Autodesk Inventor part; units mm, degrees
ref_plane "Work Plane1" through (0, 0, -15) normal (0, 0, 1) x (1, 0, 0)
ref_plane "YZ Plane" through (0, 0, 0) normal (1, 0, 0) x (0, 1, 0)
ref_plane "XZ Plane" through (0, 0, 0) normal (0, 1, 0) x (-1, 0, 0)
sketch "Sketch1" plane through (0, 0, 0) normal (0, 0, 1) x (1, 0, 0)
  line L0 (0, 0) -> (25, 0)
  line L1 (25, 0) -> (25, 40)
  line L2 (25, 40) -> (0, 40)
  line L3 (0, 40) -> (0, 0)
  dimension "d1" = 25
  dimension "d2" = 40
  dimension "d3" = 25
extrude "Extrusion1" add sketch "Sketch1" against normal blind 30
sketch "Sketch2" plane through (25, 0, 0) normal (1, 0, 0) x (0, 0, -1)
  line L0 (0, 0) -> (30, 0)
  circle A0 centre (15, 6.56) radius 2.46
extrude "Extrusion2" cut sketch "Sketch2" against normal blind 30
sketch "Sketch3" plane through (0, 0, 0) normal (-1, 0, 0) x (0, 0, 1)
  line L0 (0, 0) -> (-30, 0)
  line L1 (-25.05, 0) -> (-4.95, 0)
  line L2 (-4.95, 0) -> (-4.95, 33.12)
  line L3 (-4.95, 33.12) -> (-25.05, 33.12)
  line L4 (-25.05, 33.12) -> (-25.05, 0)
  dimension "d11" = 20.1
extrude "Extrusion3" cut sketch "Sketch3" against normal blind 20
sketch "Sketch4" plane through (0, 0, 0) normal (0, -1, 0) x (1, 0, 0)
  line L0 (20, -4.95) -> (20, -25.05)
  line L1 (20, -15) -> (25, -15)
  line L2 (25, 0) -> (25, -30)
  line L3 (20, -8.025) -> (25, -8.025)
  line L4 (25, -8.025) -> (25, -21.975)
  line L5 (25, -21.975) -> (20, -21.975)
  line L6 (20, -21.975) -> (20, -8.025)
  line L7 (20, -8.025) -> (25, -21.975) construction
  line L8 (25, -8.025) -> (20, -21.975) construction
  line L9 (25, -12.54) -> (25, -17.46)
  point P0 (0, 0)
  point P1 (22.5, -15)
  dimension "d14" = 13.95
extrude "Extrusion4" add sketch "Sketch4" along normal blind 15
sketch "Sketch5" plane through (20, 0, 0) normal (-1, 0, 0) x (0, 0, 1)
  circle A0 centre (-15, 6.56) radius 2.46
  circle A1 centre (-15, 6.56) radius 4.7025
  circle A2 centre (-15, 6.56) radius 2.46
  circle A3 centre (-15, 6.56) radius 2.46
  point P0 (0, 0)
  dimension "d17" = 9.405
extrude "Extrusion5" cut sketch "Sketch5" against normal blind 2.1
sketch "Sketch6" plane through (25, 0, 0) normal (1, 0, 0) x (0, 0, -1)
  circle A0 centre (15, 6.56) radius 4.7025
  line L0 (15, 6.56) -> (15, 23.56)
  circle A1 centre (15, 23.56) radius 2.46
  point P0 (0, 0)
  dimension "d20" = 17
  dimension "d21" = 4.92
extrude "Extrusion6" cut sketch "Sketch6" against normal blind 10 contours A1
sketch "Sketch7" plane through (20, 0, 0) normal (-1, 0, 0) x (0, 0, 1)
  circle A0 centre (-15, 23.56) radius 2.46
  circle A1 centre (-15, 23.56) radius 4.7025
  point P0 (0, 0)
  dimension "d24" = 9.405
extrude "Extrusion7" cut sketch "Sketch7" against normal blind 2.1
sketch "Sketch9" plane through (25, 0, 0) normal (1, 0, 0) x (0, 0, -1)
  circle A0 centre (15, 6.56) radius 2.46
  circle A1 centre (15, 6.56) radius 2.46
  circle A2 centre (15, 23.56) radius 2.46
  circle A3 centre (15, 23.56) radius 2.46
  line L0 (30, 40) -> (30, 0)
  line L1 (30, 0) -> (30, 40)
  line L2 (30, 40) -> (0, 40)
  line L3 (0, 40) -> (0, 0)
  line L4 (0, 0) -> (8.025, 0)
  line L5 (21.975, 0) -> (21.975, -15)
  line L6 (21.975, -15) -> (8.025, -15)
  line L7 (8.025, -15) -> (8.025, 0)
  line L8 (0, 0) -> (8.025, 0)
  line L9 (21.975, 0) -> (30, 0)
extrude "Extrusion8" add sketch "Sketch9" along normal blind 5
sketch "Sketch10" plane through (0, 40, 0) normal (0, 1, 0) x (1, 0, 0)
  line L0 (0, 30) -> (30, 30)
  line L1 (30, 0) -> (0, 0)
  line L2 (0, 30) -> (30, 30)
  line L3 (30, 30) -> (30, 0)
  line L4 (30, 0) -> (0, 0)
  line L5 (0, 0) -> (0, 30)
extrude "Extrusion9" add sketch "Sketch10" along normal blind 30
sketch "Sketch12" plane through (30, 0, 0) normal (1, 0, 0) x (0, 0, -1)
  circle A0 centre (15, 6.56) radius 2.46
  line L0 (15, 6.56) -> (15, 15.06)
  circle A1 centre (15, 15.06) radius 2.525
  point P0 (0, 0)
  dimension "d31" = 8.5
  dimension "d33" = 5.05
extrude "Extrusion10" cut sketch "Sketch12" against normal blind 30 contours A1
sketch "Sketch14" plane through (0, 0, 0) normal (0, 0, 1) x (1, 0, 0)
  line L0 (30, 70) -> (0, 70)
  line L1 (0, 70) -> (0, 85)
  line L2 (-15, 100) -> (-23, 100)
  line L3 (30, 0) -> (30, 70)
  line L4 (30, 122.5) -> (30, 70)
  arc A0 (0, 85) -> (-15, 100) centre (-15, 85) ccw
  line L5 (30, 105) -> (30, 100)
  line L6 (-23, 153) -> (15, 153)
  line L7 (-18, 150.5) -> (-23, 153)
  line L8 (-18, 102.5) -> (-23, 100)
  line L9 (-18, 102.5) -> (-13, 126.5)
  line L10 (-13, 126.5) -> (-18, 150.5)
  line L11 (30, 126.5) -> (15, 153)
  line L12 (30, 122.5) -> (30, 126.5)
  point P0 (0, 0)
  point P1 (0, 100)
  dimension "d47" = 30
  dimension "d54" = 15
extrude "Extrusion12" add sketch "Sketch14" against normal blind 30
sketch "Sketch15" plane through (0, 0, -25.05) normal (-1, 0, 0) x (0, 0, 1)
  line L0 (0, 33.12) -> (20.1, 33.12)
  line L1 (20.1, 33.12) -> (20.1, 0)
  line L2 (0, 33.12) -> (20.1, 33.12)
  line L3 (20.1, 33.12) -> (20.1, 31.1)
  line L4 (20.1, 31.1) -> (0, 31.1)
  line L5 (0, 31.1) -> (0, 33.12)
  point P0 (25.05, 0)
  dimension "d57" = 2.02
extrude "Extrusion13" add sketch "Sketch15" against normal blind 20
sketch "Sketch25" plane through (0, 0, 0) normal (0, 0, 1) x (1, 0, 0)
  line L0 (-15, 100) -> (-23, 100)
  line L1 (-15, 100) -> (-23, 100)
  line L2 (-23, 100) -> (-18, 102.5)
  line L3 (-23, 100) -> (-18, 102.5)
  line L4 (-18, 102.5) -> (-13, 126.5)
  line L5 (-18, 102.5) -> (-13, 126.5)
  line L6 (-13, 126.5) -> (-18, 150.5)
  line L7 (-13, 126.5) -> (-18, 150.5)
  line L8 (-18, 150.5) -> (-23, 153)
  line L9 (-18, 150.5) -> (-23, 153)
  line L10 (-23, 153) -> (15, 153)
  line L11 (-23, 153) -> (15, 153)
  line L12 (15, 153) -> (30, 126.5)
  line L13 (15, 153) -> (30, 126.5)
  line L14 (30, 126.5) -> (30, 76.5)
  line L15 (30, 0) -> (30, 126.5)
  line L16 (30, 76.5) -> (0, 76.5)
  arc A0 (0, 85) -> (-15, 100) centre (-15, 85) ccw
  line L17 (0, 76.5) -> (0, 85)
  line L18 (0, 85) -> (0, 0)
  arc A1 (0, 85) -> (-15, 100) centre (-15, 85) ccw
  dimension "d90" = 50
extrude "Extrusion14" add sketch "Sketch25" along normal blind 30
ref_plane "Work Plane1" through (0, 0, -15) normal (0, 0, 1) x (1, 0, 0)
mirror "Mirror1" about plane through (0, 0, -15) normal (0, 0, 1) of "Extrusion14"
properties part number "rec_a_48mm_x_90mm"
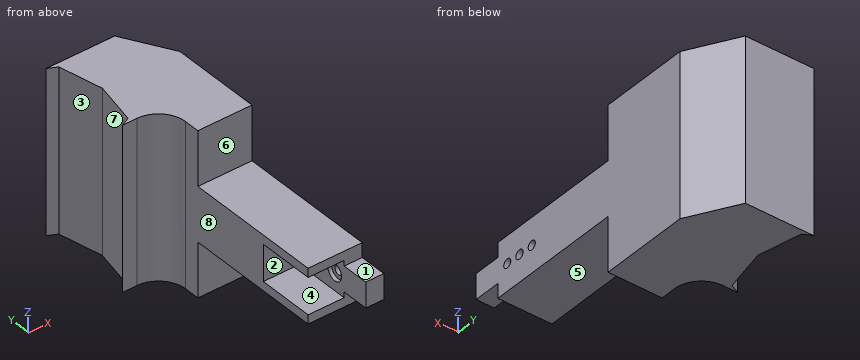
Here's how the part is built. I have some questions about the finished solid (model axes, mm). Face numbers are marked on the shaded views. A direction names the side the tool comes from. Give positions to 0.01 mm unless a question says otherwise; leave off trailing zeros. Order: outer loops, then holes, each group sorted by start corner. A loop starts at its lowest first (then second) coordinate and runs counter-clockwise, first axis right, second up. Notation, with made-up numbers: M -4,-37.75 L 11,-37.75 A22 cw 11,-18.75 Z; hole C 19.5,-18 d4. An arc over 180 degrees is marked long. Use a Markdown table: item, result. Add a question column.
1. Suppose I cut it at D-D (y = 62). List the corners of the cut face in (x, z) for me.
2. For pin 1 Ø24 at (x, z) = (18.5, -40) entering from -Y; pin 2 Ø4.5 at (y, z) = (25.5, -14.5) entering from -X; pin 3 Ø16 at (y, z) = (9, -16) entering from -X; pin 4 Ø4 at (y, z) = (15.06, -15) entering from -X, each with a flat end and sliding along its axis, tell me the tip position at first contact or that it passes through.
3. Suppose I cut it at B-B (z = -15). Give the number of separate pieces and of enclosed holes in the cut face, and give its area (3 significant figures).
4. On a 3-axis mill with a long thin cutter (end or side, diameter ignored), from which of +Z, -Z, +X, -X, +Y, -Y can I reach the whole of each face in a straight line? I mean the marked faces 4, 5, 6, 7 and 8. Say none if no direction works.
5. Suppose I cut it at A-A (y = 23.56). List the corners of the cut face in (x, z) for me, and give its area (3 significant figures).
6. I need wall thicknesses on probe 1 along Z at (x, y) = (15, 25); probe 2 along Z at (x, y) = (22.25, 15.06) (3 decimals); probe 3 along Y at (x, z) = (23.5, -15) (3 decimals). Which ranges of each line are inside material? Lowest first, please. Write a range as from..to.
7. Suppose I cut it at C-C (z = 21). List the corners of the cut face in (x, y) for me, and give its area (3 significant figures).
8. If we mould it in two halves opening along Y, with no side actions, what happens to the marked faces 1, 2 and 3? For each: +Y half, -Y half, draft (parallel to the pull), parting line (faces both ways), or undercut.
Results list:
| question | item | result |
|---|---|---|
| 1 | outline | M 0,-30 L 30,-30 L 30,0 L 0,0 Z |
| 2 | pin 1 | stops at y = 0 |
| 2 | pin 2 | stops at x = 22.1 |
| 2 | pin 3 | stops at x = 20 |
| 2 | pin 4 | passes through |
| 3 | separate pieces | 4 |
| 3 | enclosed holes | 0 |
| 3 | area | 4,650 mm² |
| 4 | face 4 | -X, -Y |
| 4 | face 5 | -Z, +X, -X, -Y |
| 4 | face 6 | +Z, +X, -X, -Y |
| 4 | face 7 | +Z, -Z, -X |
| 4 | face 8 | +Z, -Z, -X, -Y |
| 5 | outline | M 0,-30 L 30,-30 L 30,-17.46 L 22.1,-17.46 L 22.1,-19.7 L 20,-19.7 L 20,-25.05 L 0,-25.05 Z; M 0,-4.95 L 20,-4.95 L 20,-10.3 L 22.1,-10.3 L 22.1,-12.54 L 30,-12.54 L 30,0 L 0,0 Z |
| 5 | area | 439 mm² |
| 6 | probe 1 | z = -30..-25.05, -4.95..0 |
| 6 | probe 2 | z = -30..-17.525, -12.475..0 |
| 6 | probe 3 | y = -15..4.1, 9.02..12.535, 17.585..21.1, 26.02..137.983 |
| 7 | outline | M -23,100 L -15,100 A15 cw 0,85 L 0,76.5 L 30,76.5 L 30,126.5 L 15,153 L -23,153 L -18,150.5 L -13,126.5 L -18,102.5 Z |
| 7 | area | 2,990 mm² |
| 8 | face 1 | draft |
| 8 | face 2 | -Y half |
| 8 | face 3 | undercut |
